Check sheet for the modelled part. Datum: model origin and axes. Units: mm. Face numbers are marked on the shaded views. A direction names the side the tool comes from. Coordinates: 2 decimals unless noted, no trailing zeros. Loops run counter-clockwise (first coordinate to the right, second up) from the corner with the lowest first, then second, coordinate; pieces in that order, holes last. Notation, with made-up numbers: M -38.75,75 L -4.75,75 A4 cw -4.75,79 Z; hole C 59.5,-32 d8. An arc over 180 degrees is marked long. Answer as CSV lines item,"result". Start each with the question number.
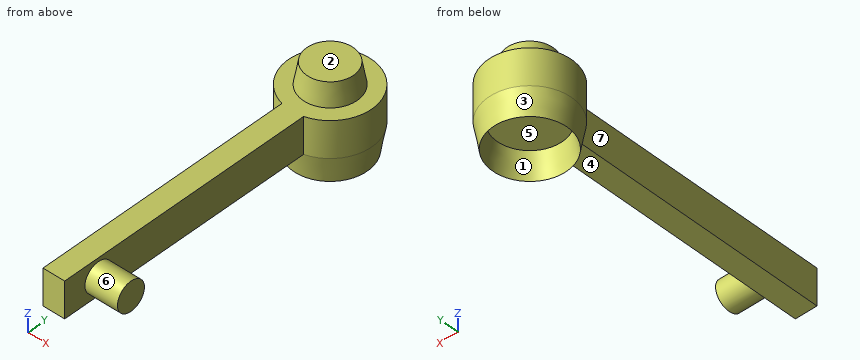
from build123d import *

# Parameters (mm, degrees)
BOSS_EXTRUDE1_DEPTH = 5
SKETCH2_R           = 7.5
BOSS_EXTRUDE2_DEPTH = 6
BOSS_EXTRUDE2_TAPER = 10
SKETCH3_R           = 4
BOSS_EXTRUDE3_DEPTH = 9
SKETCH4_R           = 11.5
SKETCH4_R_2         = 9
BOSS_EXTRUDE4_DEPTH = 9
BOSS_EXTRUDE4_TAPER = 10


with BuildPart() as part:
    # Sketch1 → Boss-Extrude1 (new, symmetric)
    with BuildSketch(Plane.XY):
        with BuildLine():
            Line((3, 29.898198344), (3, -41))
            Line((3, -41), (-3, -41))
            Line((-3, -41), (-3, 29.898198344))
            ThreePointArc((-3, 29.898198344), (0, 52.5), (3, 29.898198344))
        make_face()
    extrude(amount=BOSS_EXTRUDE1_DEPTH, both=True)

    # Sketch2 → Boss-Extrude2 (add)
    with BuildSketch(Plane.XY.offset(5)):
        with Locations((0, 41)):
            Circle(SKETCH2_R)
    extrude(amount=BOSS_EXTRUDE2_DEPTH, taper=BOSS_EXTRUDE2_TAPER)

    # Sketch3 → Boss-Extrude3 (add)
    with BuildSketch(Plane(origin=(3, 0, 0), x_dir=(0, 0, -1), z_dir=(1, 0, 0))):
        with Locations(Location((0, -31, 0), (0, 0, 90))):
            Circle(SKETCH3_R)
    extrude(amount=BOSS_EXTRUDE3_DEPTH)

    # Sketch4 → Boss-Extrude4 (add)
    with BuildSketch(Plane(origin=(0, 0, -5), x_dir=(-1, 0, 0), z_dir=(0, 0, -1))):
        with Locations((0, 41)):
            Circle(SKETCH4_R)
        with Locations((0, 41)):
            Circle(SKETCH4_R_2, mode=Mode.SUBTRACT)
    extrude(amount=BOSS_EXTRUDE4_DEPTH, taper=BOSS_EXTRUDE4_TAPER)


solid = part.part
Item 1: Sectioned sample at A-A, the plane y = -31. Record the boundary of the cut face in (x, z).
Item 2: Go/stop test with flat-tipped pins: pin 1 (2 mm diameter, centred on x = -2, y = 17.5, fed in from -Z); pin 2 (5 mm diameter, centred on y = 0.5, z = 1, fed in from -X); pin 3 (3 mm diameter, centred on x = -4.5, z = 8.5, fed in from +Y). Record where each tip stops, or that it passes through.
Item 3: Material ranges on line 1 (X direction, y = -32, z = 1.5); line 2 (X direction, y = 23, z = -2.5); line 3 (Z direction, x = -2.25, y = -15), recorded low to high. Write a range as from..to.
Item 4: Sectioned sample at D-D, the plane y = -1. Record the boundary of the cut face in (x, z).
Item 5: Sectioned sample at C-C, the plane z = 0. Record the boundary of the cut face in (x, y), and give its area (3 significant figures).
Item 6: Set-up check for the marked faces 4, 5, 6 and 7: record each of +Z, -Z, +X, -X, +Y, -Y from which the full face is reachable in a straight line by a thin tool's end or side.
Item 7: Release check for a two-part mould opening along X. For the marked faces 1, 2 and 3 record: released by +X, released by -X, zero draft, split by the parting line, or undercut.
Item 8: Sectioned sample at B-B, the plane x = 0. Record the boundary of the cut face in (y, z), and give its area (3 significant figures).
Reply:
1,outline,"M -3,-5 L 3,-5 L 3,-4 L 12,-4 L 12,4 L 3,4 L 3,5 L -3,5 Z"
2,pin 1,"z = -5"
2,pin 2,"x = -3"
2,pin 3,"y = 47.25"
3,line 1,"-3..12"
3,line 2,"-3..3"
3,line 3,"-5..5"
4,outline,"M -3,-5 L 3,-5 L 3,5 L -3,5 Z"
5,outline,"M -3,-41 L 3,-41 L 3,-35 L 12,-35 L 12,-27 L 3,-27 L 3,29.9 A11.5 ccw long -3,29.9 Z"
5,area,"911 mm²"
6,face 4,"-Z, +X, -X, -Y"
6,face 5,"-Z"
6,face 6,"+X"
6,face 7,"+Z, -Z, -X, -Y"
7,face 1,"undercut"
7,face 2,"zero draft"
7,face 3,"split by the parting line"
8,outline,"M -41,-5 L 29.5,-5 L 30.75,-12.09 L 32,-5 L 50,-5 L 51.25,-12.09 L 52.5,-5 L 52.5,5 L 48.5,5 L 47.44,11 L 34.56,11 L 33.5,5 L -41,5 Z"
8,area,"1,040 mm²"
